from build123d import *

# Parameters (mm, degrees)
SKETCH1_W           = 60
SKETCH1_H           = 84
RAIL_PLATE_DEPTH    = 6
DOVETAIL_RAIL_DEPTH = 72
SKETCH3_R           = 1.7
M3_HOLES_DEPTH      = 7
SKETCH4_R           = 3
COUNTERBORES_DEPTH  = 4
SKETCH5_R           = 2.25
LOCK_DETENTS_DEPTH  = 2.5


with BuildPart() as part:
    # Sketch1 → Rail Plate (new body)
    with BuildSketch(Plane(origin=(0, -34.4, 0), x_dir=(1, 0, 0), z_dir=(0, 1, 0))):
        with Locations((0, -70)):
            Rectangle(SKETCH1_W, SKETCH1_H)
    extrude(amount=RAIL_PLATE_DEPTH)

    # Sketch2 → Dovetail Rail (add)
    with BuildSketch(Plane.XY.offset(34)):
        Polygon((-14.666666667, -33.9), (14.666666667, -33.9), (19, -40.4), (-19, -40.4), align=None)
    extrude(amount=DOVETAIL_RAIL_DEPTH)

    # Sketch3 → M3 Holes (cut)
    with BuildSketch(Plane(origin=(0, -34.9, 0), x_dir=(1, 0, 0), z_dir=(0, 1, 0))):
        with Locations(Location((-22, -91, 0), (0, 0, 270))):
            Circle(SKETCH3_R)
        with Locations(Location((-22, -49, 0), (0, 0, 270))):
            Circle(SKETCH3_R)
        with Locations(Location((22, -91, 0), (0, 0, 270))):
            Circle(SKETCH3_R)
        with Locations(Location((22, -49, 0), (0, 0, 270))):
            Circle(SKETCH3_R)
    extrude(amount=M3_HOLES_DEPTH, mode=Mode.SUBTRACT)

    # Sketch4 → Counterbores (cut)
    with BuildSketch(Plane(origin=(0, -34.9, 0), x_dir=(1, 0, 0), z_dir=(0, 1, 0))):
        with Locations(Location((-22, -91, 0), (0, 0, 270))):
            Circle(SKETCH4_R)
        with Locations(Location((-22, -49, 0), (0, 0, 270))):
            Circle(SKETCH4_R)
        with Locations(Location((22, -91, 0), (0, 0, 270))):
            Circle(SKETCH4_R)
        with Locations(Location((22, -49, 0), (0, 0, 270))):
            Circle(SKETCH4_R)
    extrude(amount=COUNTERBORES_DEPTH, mode=Mode.SUBTRACT)

    # Sketch5 → Lock Detents (cut)
    with BuildSketch(Plane(origin=(0, -40.9, 0), x_dir=(1, 0, 0), z_dir=(0, 1, 0))):
        with Locations(Location((0, -98, 0), (0, 0, 270))):
            Circle(SKETCH5_R)
        with Locations(Location((0, -42, 0), (0, 0, 270))):
            Circle(SKETCH5_R)
    extrude(amount=LOCK_DETENTS_DEPTH, mode=Mode.SUBTRACT)


solid = part.part
Build history of the part. All positions in model axes, mm. A direction names the side the tool comes from. Round coordinates to 2 decimals unless told otherwise and drop trailing zeros. Loops run counter-clockwise (first coordinate to the right, second up) from the corner with the lowest first, then second, coordinate; pieces in that order, holes last. Notation, with made-up numbers: (9, -31.5) -> (30, -31.5) arc R14 ccw to (30, -13.5) -> close; hole circle Ø4 at (-40, -27). An arc over 180 degrees is marked (long way). One line per item, written item: value. Start each with the question number.
Q1. Cut at A-A on x = -17. List the corners of the cut face in (y, z).
Q2. Drop flat-ended pins along their axis: pin 1 Ø1.3 at (x, z) = (-1, 42.5) entering from -Y; pin 2 Ø1.8 at (x, z) = (-22.5, 90) entering from -Y; pin 3 Ø1.8 at (x, y) = (-7.5, -38.5) entering from -Z. Give the stop position or say it passes through.
Q3. Two-plate mould, pull along Z, no slides. Class faces 1 (the face through (0, -31, 112)), 2 (the face through (22.07, -29.67, 89.3)), 3 (the face through (0, -28.4, 69)), 4 (the face through (0, -37, 34)): released by +Z, released by -Z, zero draft, split by the parting line, or undercut.
Q4. Cut at D-D on y = -33. List the corners of the cut face in (x, z).
Q5. 3-axis set-ups, long thin cutter, end or side, ignore diameter. For faces 5 (the face through (0, -40.4, 69)), 6 (the face through (0, -37, 106)), 7 (the face through (17, -37.4, 69.5)), 8 (the face through (-22, -33, 88)), 9 (the face through (-17, -37.4, 69.5)): which of +Z, -Z, +X, -X, +Y, -Y reach the whole face in a straight line?
Q6. Cut at B-B on z = 49. List the corners of the cut face in (x, y).
Q7. Probe line 1 along X through (y, z) = (-32.9, 91); line 2 along X through (y, z) = (-30.05, 91); line 3 along Z through (x, y) = (-22, -32.4). List the from-to ranges inside material, lowest first.
Q8. Cut at C-C on z = 98. List the corners of the cut face in (x, y).
Computed:
1. outline: (-40.4, 34) -> (-37.4, 34) -> (-37.4, 106) -> (-40.4, 106) -> close; (-34.4, 28) -> (-28.4, 28) -> (-28.4, 112) -> (-34.4, 112) -> close
2. pin 1: y = -38.4
2. pin 2: y = -30.9
2. pin 3: z = 34
3. face 1: released by +Z
3. face 2: undercut
3. face 3: zero draft
3. face 4: released by -Z
4. outline: (-30, 28) -> (30, 28) -> (30, 112) -> (-30, 112) -> close; hole circle Ø6 at (-22, 49); hole circle Ø6 at (-22, 91); hole circle Ø6 at (22, 49); hole circle Ø6 at (22, 91)
5. face 5: +Z, -Z, +X, -X, -Y
5. face 6: +Z, +X, -X, -Y
5. face 7: +Z, -Z, +X
5. face 8: -Y
5. face 9: +Z, -Z, -X
6. outline: (-30, -34.4) -> (-25, -34.4) -> (-25, -30.9) -> (-23.7, -30.9) -> (-23.7, -28.4) -> (-30, -28.4) -> close; (-20.3, -30.9) -> (-19, -30.9) -> (-19, -34.4) -> (-15, -34.4) -> (-19, -40.4) -> (19, -40.4) -> (15, -34.4) -> (19, -34.4) -> (19, -30.9) -> (20.3, -30.9) -> (20.3, -28.4) -> (-20.3, -28.4) -> close; (23.7, -30.9) -> (25, -30.9) -> (25, -34.4) -> (30, -34.4) -> (30, -28.4) -> (23.7, -28.4) -> close
7. line 1: -30 to -25, -19 to 19, 25 to 30
7. line 2: -30 to -23.7, -20.3 to 20.3, 23.7 to 30
7. line 3: 28 to 46, 52 to 88, 94 to 112
8. outline: (-30, -34.4) -> (-15, -34.4) -> (-19, -40.4) -> (-2.25, -40.4) -> (-2.25, -38.4) -> (2.25, -38.4) -> (2.25, -40.4) -> (19, -40.4) -> (15, -34.4) -> (30, -34.4) -> (30, -28.4) -> (-30, -28.4) -> close
